Work out the finished part from the listing and answer in its coordinate system (mm). A direction names the side the tool comes from. Coordinates: 2 decimals unless noted, no trailing zeros. Write each loop counter-clockwise with the first axis right and the second up, starting at its lowest first coordinate (ties: lowest second). Pieces come first, ordered by that corner, then holes. Notation, with made-up numbers: (31, 48) -> (82, 48) arc R20 cw to (82, 72) -> close; hole circle Ø3 at (73.25, -12). An arc over 180 degrees is marked (long way). Write each question's results on one line, items separated by ' | '. Start each with the question number.
from build123d import *

# Parameters (mm, degrees)
BOSS_EXTRUDE1_DEPTH             = 20
CUT_EXTRUDE1_DEPTH              = 45
M6X1_0_TAPPED_HOLE1_D           = 5
M6X1_0_TAPPED_HOLE1_DEPTH       = 15
M6X1_0_TAPPED_HOLE1_CSINK_D     = 6.05
M6X1_0_TAPPED_HOLE1_CSINK_ANGLE = 90
M6X1_0_TAPPED_HOLE1_TIP         = 1.502151548


with BuildPart() as part:
    # Sketch1 → Boss-Extrude1 (new body)
    with BuildSketch(Plane.XY):
        Polygon((6.5, 0), (-6.5, 0), (-9.8, 2), (-9.8, 5.5), (-4.9, 5.5), (-4.9, 10.5), (4.9, 10.5), (4.9, 5.5), (9.8, 5.5), (9.8, 2), align=None)
    extrude(amount=-BOSS_EXTRUDE1_DEPTH)

    # Sketch2 → Cut-Extrude1 (cut)
    with BuildSketch(Plane.XY):
        Polygon((-0.9, 10.5), (0, 9.6), (0.9, 10.5), align=None)
    extrude(amount=-CUT_EXTRUDE1_DEPTH, mode=Mode.SUBTRACT)

    # M6x1.0 Tapped Hole1
    with Locations(Plane(origin=(0, 10.5, 0), x_dir=(1, 0, 0), z_dir=(0, 1, 0))):
        with Locations((0, 10)):
            CounterSinkHole(M6X1_0_TAPPED_HOLE1_D / 2, M6X1_0_TAPPED_HOLE1_CSINK_D / 2, depth=M6X1_0_TAPPED_HOLE1_DEPTH, counter_sink_angle=M6X1_0_TAPPED_HOLE1_CSINK_ANGLE)
            with Locations((0, 0, -(M6X1_0_TAPPED_HOLE1_DEPTH + M6X1_0_TAPPED_HOLE1_TIP / 2))):  # 118° drill point
                Cone(0, M6X1_0_TAPPED_HOLE1_D / 2, M6X1_0_TAPPED_HOLE1_TIP, mode=Mode.SUBTRACT)


solid = part.part
1. Given pin 1 Ø4 at (x, z) = (-8, -11) entering from +Y; pin 2 Ø4 at (y, z) = (8, -13) entering from +X, each flat-ended and moving along its own axis, determine where each tip first touches the part or whether it passes through.
2. Find section B-B on y = 1. Give the vertices of the cut face in (x, z).
3. Find section D-D on x = -6. Give the vertices of the cut face in (y, z), and give its area (3 significant figures).
4. Find section C-C on z = -3. Give the vertices of the cut face in (x, y).
5. Determine the mould class of faces 4 (the face through (0.4, 10, -16.2)), 5 (the face through (0, 4, 0)), 6 (the face through (2.642, 10.117, -10.053)) for opening direction Z: pulls with the +Z half, pulls with the -Z half, needs draft (parallel to the pull), parting line crosses it, or undercut.
6. Find section A-A on z = -10. Give the vertices of the cut face in (x, y) (3 decimals), and give its area (3 significant figures).
7. Find the intervals of material crossed by L1, parallel to X at y = 3.75, z = -10; L2, parallel to Z at x = 0, y = 3.5; L3, parallel to X at y = 7, z = -10, in increasing order.
8. For faces 1 (the face through (4.9, 8, -10)), 2 (the face through (0.4, 10, -3.7)), 3 (the face through (-4.9, 8, -10)), determine the directions among +Z, -Z, +X, -X, +Y, -Y from which every point of the face is accessible in a straight line to the end or side of a thin tool.
Ans:
1) pin 1: stops at y = 5.5 | pin 2: stops at x = 4.9
2) outline: (-8.15, -20) -> (8.15, -20) -> (8.15, 0) -> (-8.15, 0) -> close; hole circle Ø5 at (0, -10)
3) outline: (0, -20) -> (5.5, -20) -> (5.5, 0) -> (0, 0) -> close | area: 110 mm²
4) outline: (-9.8, 2) -> (-6.5, 0) -> (6.5, 0) -> (9.8, 2) -> (9.8, 5.5) -> (4.9, 5.5) -> (4.9, 10.5) -> (0.9, 10.5) -> (0, 9.6) -> (-0.9, 10.5) -> (-4.9, 10.5) -> (-4.9, 5.5) -> (-9.8, 5.5) -> close
5) face 4: needs draft | face 5: pulls with the +Z half | face 6: undercut
6) outline: (-9.8, 2) -> (-6.5, 0) -> (-2.5, 0) -> (-2.5, 9.975) -> (-3.025, 10.5) -> (-4.9, 10.5) -> (-4.9, 5.5) -> (-9.8, 5.5) -> close; (2.5, 0) -> (6.5, 0) -> (9.8, 2) -> (9.8, 5.5) -> (4.9, 5.5) -> (4.9, 10.5) -> (3.025, 10.5) -> (2.5, 9.975) -> close | area: 97.4 mm²
7) L1: x = -9.8 to -2.5, 2.5 to 9.8 | L2: z = -20 to -12.5, -7.5 to 0 | L3: x = -4.9 to -2.5, 2.5 to 4.9
8) face 1: +Z, -Z, +X, +Y | face 2: +Z, -Z, +Y | face 3: +Z, -Z, -X, +Y
